Check sheet for the modelled part. Datum: model origin and axes. Units: mm. A direction names the side the tool comes from. Give positions to 0.01 mm unless a question says otherwise; leave off trailing zeros. Loops run counter-clockwise (first coordinate to the right, second up) from the corner with the lowest first, then second, coordinate; pieces in that order, holes last.
```python
from build123d import *

# Parameters (mm, degrees)
ESQUISSE1_W             = 30.48
ESQUISSE1_H             = 12.7
BOSS_EXTRU_1_DEPTH      = 0.7
CONG_1_R                = 0.5
ESQUISSE2_R             = 1.5
ENL_V_MAT_EXTRU_1_DEPTH = 1.7
BOSS_EXTRU_2_DEPTH      = 6
CONG_2_R                = 1
BOSS_EXTRU_3_DEPTH      = 5
CONG_3_R                = 1


with BuildPart() as part:
    # Esquisse1 → Boss.-Extru.1 (new body)
    with BuildSketch(Plane.XY):
        Rectangle(ESQUISSE1_W, ESQUISSE1_H)
    extrude(amount=BOSS_EXTRU_1_DEPTH)

    # Congé1
    cong_1_edges = [part.edges().sort_by_distance(p)[0] for p in [
        (-15.24, 6.35, 0.35),
        (15.24, 6.35, 0.35),
        (15.24, -6.35, 0.35),
        (-15.24, -6.35, 0.35),
    ]]
    fillet(cong_1_edges, radius=CONG_1_R)

    # Esquisse2 → Enlèv. mat.-Extru.1 (cut, through all)
    with BuildSketch(Plane.XY.offset(0.7)):
        with Locations((-12.7, 0)):
            Circle(ESQUISSE2_R)
        with Locations((12.7, 0)):
            Circle(ESQUISSE2_R)
    extrude(amount=-ENL_V_MAT_EXTRU_1_DEPTH, mode=Mode.SUBTRACT)

    # Esquisse3 → Boss.-Extru.2 (add)
    with BuildSketch(Plane.XY.offset(0.7)):
        Polygon((-8.25, 3.81), (8.25, 3.81), (7, -3.81), (-7, -3.81), align=None)
    extrude(amount=BOSS_EXTRU_2_DEPTH)

    # Congé2
    cong_2_edges = [part.edges().sort_by_distance(p)[0] for p in [
        (-8.25, 3.81, 3.7),
        (-7, -3.81, 3.7),
        (7, -3.81, 3.7),
        (8.25, 3.81, 3.7),
    ]]
    fillet(cong_2_edges, radius=CONG_2_R)

    # Esquisse4 → Boss.-Extru.3 (add)
    with BuildSketch(Plane(origin=(0, 0, 0), x_dir=(-1, 0, 0), z_dir=(0, 0, -1))):
        Polygon((-9.5, 5.3), (9.5, 5.3), (8.25, -5.3), (-8.25, -5.3), align=None)
    extrude(amount=BOSS_EXTRU_3_DEPTH)

    # Congé3
    cong_3_edges = [part.edges().sort_by_distance(p)[0] for p in [
        (9.5, 5.3, -2.5),
        (8.25, -5.3, -2.5),
        (-8.25, -5.3, -2.5),
        (-9.5, 5.3, -2.5),
    ]]
    fillet(cong_3_edges, radius=CONG_3_R)


solid = part.part
```
(1) Section check D-D on y = 0. Record the boundary of the cut face in (x, z) (3 decimals), plus the area to 3 significant figures.
(2) Access from +Z, -Z, +X, -X, +Y, -Y to the whole of each face (thin tool, end or side, straight path). Record for faces 1 (the face through (-8.033, -5.041, -2.535)), 2 (the face through (0, 4, 0.7)), 3 (the face through (6.79, -3.58, 3.74)).
(3) Gauge pin test, flat ends, axial feed: pin 1 Ø2.5 at (x, y) = (-12.7, 0) entering from -Z; pin 2 Ø5 at (x, z) = (-7, 4.5) entering from +Y; pin 3 Ø1.5 at (x, y) = (-10, -3.5) entering from +Z; pin 4 Ø4 at (x, z) = (-1, -2.5) entering from -Y. Record the tip position at first contact, or that the pin passes through.
(4) Material ranges on line 1 (Y direction, x = 12.7, z = 0.4); line 2 (Z direction, x = -3.5, y = -4); line 3 (Z direction, x = -11, y = -0.25), recorded low to high.
(5) Section check B-B on z = -2.5. Record the boundary of the cut face in (x, y), plus the area to 3 significant figures.
(6) Release check for a two-part mould opening along Y. For faces 4 (the face through (-11.314, -0.575, 0.355)), 5 (the face through (0, 5.3, -2)), 6 (the face through (-6.806, -3.566, 3.742)) record: pulls with the +Y half, pulls with the -Y half, needs draft (parallel to the pull), parting line crosses it, or undercut.
(7) Section check A-A on x = -12.7. Record the boundary of the cut face in (y, z).
(8) Section check C-C on x = 1. Record the boundary of the cut face in (y, z).
Computed values:
1. outline: (-15.24, 0) - (-14.2, 0) - (-14.2, 0.7) - (-15.24, 0.7) - close; (-11.2, 0) - (-8.875, 0) - (-8.875, -5) - (8.875, -5) - (8.875, 0) - (11.2, 0) - (11.2, 0.7) - (7.625, 0.7) - (7.625, 6.7) - (-7.625, 6.7) - (-7.625, 0.7) - (-11.2, 0.7) - close; (14.2, 0) - (15.24, 0) - (15.24, 0.7) - (14.2, 0.7) - close
1. area: 197 mm2
2. face 1: -Z, -X, -Y
2. face 2: +Z
2. face 3: +Z, +X, -Y
3. pin 1: passes through
3. pin 2: stops at y = 3.81
3. pin 3: stops at z = 0.7
3. pin 4: stops at y = -5.3
4. line 1: y = -6.35 to -1.5, 1.5 to 6.35
4. line 2: z = -5 to 0.7
4. line 3: z = 0 to 0.7
5. outline: (-9.37, 4.18) - (-8.35, -4.42) arc R1 ccw to (-7.36, -5.3) - (7.36, -5.3) arc R1 ccw to (8.35, -4.42) - (9.37, 4.18) arc R1 ccw to (8.38, 5.3) - (-8.38, 5.3) arc R1 ccw to start
5. area: 187 mm2
6. face 4: undercut
6. face 5: pulls with the +Y half
6. face 6: pulls with the -Y half
7. outline: (-6.35, 0) - (-1.5, 0) - (-1.5, 0.7) - (-6.35, 0.7) - close; (1.5, 0) - (6.35, 0) - (6.35, 0.7) - (1.5, 0.7) - close
8. outline: (-6.35, 0) - (-5.3, 0) - (-5.3, -5) - (5.3, -5) - (5.3, 0) - (6.35, 0) - (6.35, 0.7) - (3.81, 0.7) - (3.81, 6.7) - (-3.81, 6.7) - (-3.81, 0.7) - (-6.35, 0.7) - close
